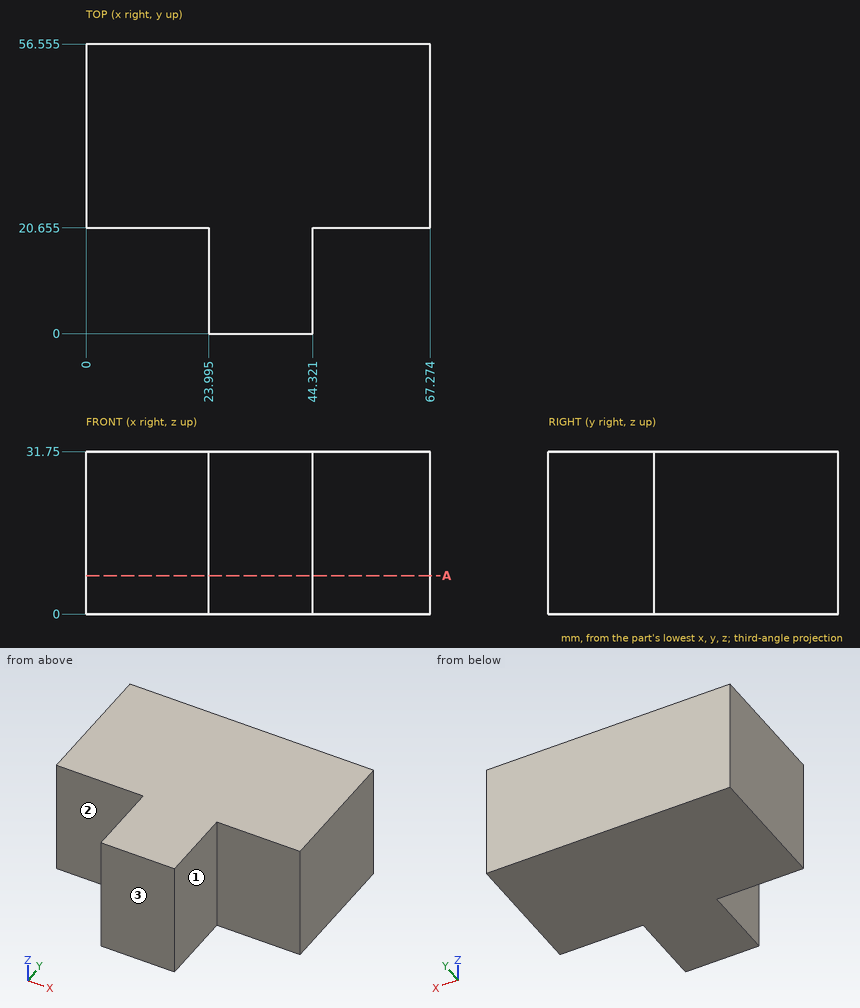
For this review, use the dimensioned drawing (mm, ordinates from the lowest corner) and the shaded views. A direction names the side the tool comes from. Coordinates: 2 decimals unless noted, no trailing zeros. Order: outer loops, then holes, each group sorted by start corner. A loop starts at its lowest first (then second) coordinate and runs counter-clockwise, first axis right, second up. Notation, with made-up numbers: M 19.25,59 L 40.25,59 A21 cw 40.25,63 Z; hole C 58.5,24 d1. An arc over 180 degrees is marked long. Answer as a JSON object with one key per item and string values. Group by question number.
1) Add section A-A, the plane z = 7.5. Write out the cut boundary in (x, y) (1 decimal), then the cut area to 4 significant figures.
2) Tool access review of the marked faces 1, 2 and 3: name each direction out of +Z, -Z, +X, -X, +Y, -Y from which nothing blocks a thin tool from reaching the whole face with its end or side.
3) Wall thickness on L1, parallel to X at y = 7, z = 30 (1 decimal); L2, parallel to Y at x = 46, z = 9.5 (1 decimal): over which ranges is each line inside the solid? List them lowest first.
4) For pin 1 (10 mm diameter, centred on y = 14, z = 15, fed in from +X); pin 2 (7 mm diameter, centred on x = 53.5, z = 9.5, fed in from -Y) (3 decimals); pin 3 (12 mm diameter, centred on y = 14, z = 20.5, fed in from -X) (1 decimal), all flat-tipped, find the tip position at first contact; note any pin that passes through.
Computed values:
{
 "1": {"outline": "M 0,20.7 L 24,20.7 L 24,0 L 44.3,0 L 44.3,20.7 L 67.3,20.7 L 67.3,56.6 L 0,56.6 Z", "area": "2,835 mm^2"},
 "2": {"face 1": "+Z, -Z, +X, -Y", "face 2": "+Z, -Z, -X, -Y", "face 3": "+Z, -Z, +X, -X, -Y"},
 "3": {"L1": "x = 24 to 44.3", "L2": "y = 20.7 to 56.6"},
 "4": {"pin 1": "stops at x = 44.32", "pin 2": "stops at y = 20.655", "pin 3": "stops at x = 24"}
}
